Can you work these out from the model? Positions are in its coordinate system, mm. Face numbers are marked on the shaded views. A direction names the side the tool comes from. Round coordinates to 2 decimals unless told otherwise and drop trailing zeros. Write each loop counter-clockwise with the first axis right and the second up, starting at its lowest first coordinate (ties: lowest second). Pieces come first, ordered by that corner, then holes. Notation, with made-up numbers: M 0,-24.5 L 30,-24.5 A27 ccw 30,-5.5 Z; hole C -2,2 d10. An arc over 180 degrees is marked long. Answer in a Markdown table with one row per item. Add a question column.
(1) Suppose I cut it at B-B, the plane z = -11.5. Write out the boundary of the cut face in (x, y), then the cut area to 3 significant figures.
(2) If we mould it in two halves opening along X, with no side actions, what happens to the marked faces 1, 2 and 3? For each: released by +X, released by -X, zero draft, split by the parting line, or undercut.
(3) If I drill on probe 1 along X at (y, z) = (20, -10.5); probe 2 along Y at (x, z) = (36, -3.5), over which ranges is the centre line in solid material (lowest first)?
(4) I'm going to push a flat-ended pin straight in: pin 1 (3 mm diameter, centred on x = 5, z = -10, fed in from +Y). Where does the tip first touch, or does it pass through?
(5) Suppose I cut it at C-C, the plane x = 26.5. Write out the boundary of the cut face in (y, z), then the cut area to 3 significant figures.
(6) For the marked faces 4 and 5, which set-ups out of +Z, -Z, +X, -X, +Y, -Y let a thin tool reach every point of the face, with its end or its side?
(7) Suppose I cut it at A-A, the plane y = 2.5. Write out the boundary of the cut face in (x, z), then the cut area to 3 significant figures.
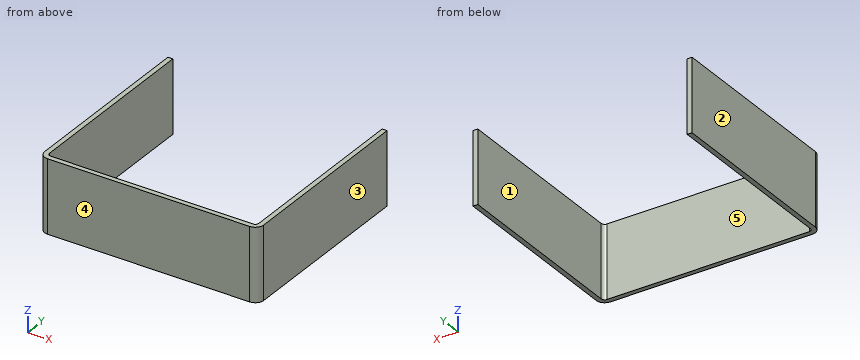
from build123d import *

# Parameters (mm, degrees)
SKETCH_1_W                       = 45
SKETCH_1_H                       = 15
SM_BASE_FLANGE_1_DEPTH           = 1
SM_EDGE_FLANGE_1_STRIP_W         = 5.4732
SM_EDGE_FLANGE_1_STRIP_H         = 1
SM_EDGE_FLANGE_1_STRIP_CUT_DEPTH = 15
SM_EDGE_FLANGE_1_DEPTH           = 15
SM_EDGE_FLANGE_2_STRIP_W         = 5.4732
SM_EDGE_FLANGE_2_STRIP_H         = 1
SM_EDGE_FLANGE_2_STRIP_CUT_DEPTH = 15
SM_EDGE_FLANGE_2_DEPTH           = 15


# Sheet-metal steps are written as plain solids
with BuildPart() as part:
    # Sketch 1 → Базовая кромка1 (new body)
    with BuildSketch(Plane(origin=(0, 0, 0), x_dir=(1, 0, 0), z_dir=(0, 1, 0))):
        with Locations((22.5, 7.5)):
            Rectangle(SKETCH_1_W, SKETCH_1_H)
    extrude(amount=-SM_BASE_FLANGE_1_DEPTH)

    # Ребро-кромка1 strip (across the edge) → Ребро-кромка1 strip cut (cut)
    with BuildSketch(Plane.XY.offset(-15)):
        with Locations((-1, -0.5)):
            Rectangle(SM_EDGE_FLANGE_1_STRIP_W, SM_EDGE_FLANGE_1_STRIP_H)
    extrude(amount=SM_EDGE_FLANGE_1_STRIP_CUT_DEPTH, mode=Mode.SUBTRACT)

    # Ребро-кромка1 section (across the edge) → Ребро-кромка1 (add)
    with BuildSketch(Plane.XY.offset(-15)):
        with BuildLine():
            Line((0, 0.7366), (0, 39))
            Line((0, 39), (1, 39))
            Line((1, 39), (1, 0.7366))
            ThreePointArc((1, 0.7366), (1.215745145, 0.215745145), (1.7366, 0))
            Line((1.7366, 0), (1.7366, -1))
            ThreePointArc((1.7366, -1), (0.508638364, -0.491361636), (0, 0.7366))
        make_face()
    extrude(amount=SM_EDGE_FLANGE_1_DEPTH)

    # Ребро-кромка2 strip (across the edge) → Ребро-кромка2 strip cut (cut)
    with BuildSketch(Plane(origin=(45, 0, 0), x_dir=(-1, 0, 0), z_dir=(0, 0, -1))):
        with Locations((-1, -0.5)):
            Rectangle(SM_EDGE_FLANGE_2_STRIP_W, SM_EDGE_FLANGE_2_STRIP_H)
    extrude(amount=SM_EDGE_FLANGE_2_STRIP_CUT_DEPTH, mode=Mode.SUBTRACT)

    # Ребро-кромка2 section (across the edge) → Ребро-кромка2 (add)
    with BuildSketch(Plane(origin=(45, 0, 0), x_dir=(-1, 0, 0), z_dir=(0, 0, -1))):
        with BuildLine():
            Line((0, 0.7366), (0, 39))
            Line((0, 39), (1, 39))
            Line((1, 39), (1, 0.7366))
            ThreePointArc((1, 0.7366), (1.215745145, 0.215745145), (1.7366, 0))
            Line((1.7366, 0), (1.7366, -1))
            ThreePointArc((1.7366, -1), (0.508638364, -0.491361636), (0, 0.7366))
        make_face()
    extrude(amount=SM_EDGE_FLANGE_2_DEPTH)


solid = part.part
Calculated:
| question | item | result |
|---|---|---|
| 1 | outline | M 0,0.74 A1.74 ccw 1.74,-1 L 43.26,-1 A1.74 ccw 45,0.74 L 45,39 L 44,39 L 44,0.74 A0.74 cw 43.26,0 L 1.74,0 A0.74 cw 1,0.74 L 1,39 L 0,39 Z |
| 1 | area | 122 mm² |
| 2 | face 1 | undercut |
| 2 | face 2 | released by -X |
| 2 | face 3 | released by +X |
| 3 | probe 1 | 0 to 1, 44 to 45 |
| 3 | probe 2 | -1 to 0 |
| 4 | pin 1 | y = 0 |
| 5 | outline | M -1,-15 L 0,-15 L 0,0 L -1,0 Z |
| 5 | area | 15.0 mm² |
| 6 | face 4 | +Z, -Z, +X, -X, -Y |
| 6 | face 5 | +Z, -Z, +Y |
| 7 | outline | M 0,-15 L 1,-15 L 1,0 L 0,0 Z; M 44,-15 L 45,-15 L 45,0 L 44,0 Z |
| 7 | area | 30.0 mm² |
